Work out the finished part from the listing and answer in its coordinate system (mm). Face numbers are marked on the shaded views. A direction names the side the tool comes from. Give positions to 0.01 mm unless a question says otherwise; leave off trailing zeros. Loops run counter-clockwise (first coordinate to the right, second up) from the corner with the lowest first, then second, coordinate; pieces in that order, holes last. Notation, with made-up numbers: (75.25, 65.25) - (125.25, 65.25) arc R33 cw to (125.25, 100.25) - close; hole circle Ø8 at (38.5, -7.75). An arc over 180 degrees is marked (long way). One line per item, written item: value.
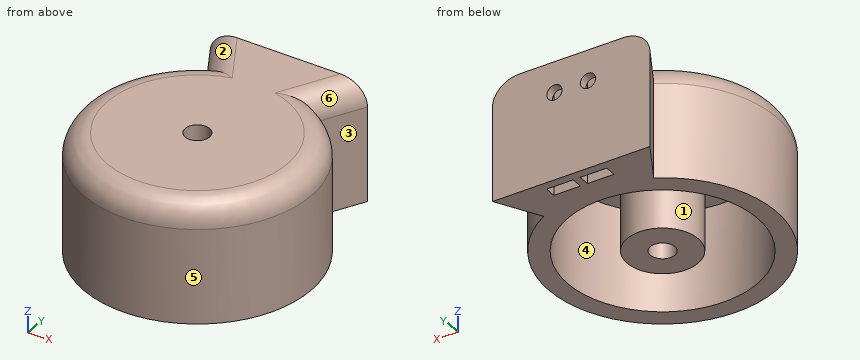
from build123d import *

# Parameters (mm, degrees)
BOSS_EXTRUDE1_DEPTH = 25
FILLET1_R           = 5
SKETCH2_R           = 2.6
CUT_EXTRUDE1_DEPTH  = 46.836666718
SKETCH4_R           = 20
SKETCH4_R_2         = 7.5
CUT_EXTRUDE2_DEPTH  = 21
CUT_EXTRUDE3_START  = 30
SKETCH5_R           = 1.6
CUT_EXTRUDE3_DEPTH  = 6
SKETCH6_W           = 5.6
SKETCH6_H           = 2.4
CUT_EXTRUDE4_DEPTH  = 22.5


with BuildPart() as part:
    # Sketch1 → Boss-Extrude1 (new body)
    with BuildSketch(Plane.XY):
        with BuildLine():
            Line((-16.642519968, 30), (16.642519968, 30))
            Line((16.642519968, 30), (11.642519968, 20.986941864))
            ThreePointArc((11.642519968, 20.986941864), (0, -24), (-11.642519968, 20.986941864))
            Line((-11.642519968, 20.986941864), (-16.642519968, 30))
        make_face()
    extrude(amount=BOSS_EXTRUDE1_DEPTH)

    # Fillet1
    fillet1_edges = [part.edges().sort_by_distance(p)[0] for p in [
        (-14.142519968, 25.493470932, 25),
    ]]
    fillet(fillet1_edges, radius=FILLET1_R)
    fillet1_2_edges = [part.edges().sort_by_distance(p)[0] for p in [
        (14.142519968, 25.493470932, 25),
    ]]
    fillet(fillet1_2_edges, radius=FILLET1_R)
    fillet1_3_edges = [part.edges().sort_by_distance(p)[0] for p in [
        (0, -24, 25),
    ]]
    fillet(fillet1_3_edges, radius=FILLET1_R - 0.0001)  # a hair under: the kernel refuses the full size

    # Sketch2 → Cut-Extrude1 (cut, through all)
    with BuildSketch(Plane.XY):
        Circle(SKETCH2_R)
    extrude(amount=CUT_EXTRUDE1_DEPTH, mode=Mode.SUBTRACT)

    # Sketch4 → Cut-Extrude2 (cut)
    with BuildSketch(Plane.XY):
        with Locations(Location((0, 0, 0), (0, 0, 180))):
            Circle(SKETCH4_R)
        with Locations(Location((0, 0, 0), (0, 0, 180))):
            Circle(SKETCH4_R_2, mode=Mode.SUBTRACT)
    extrude(amount=CUT_EXTRUDE2_DEPTH, mode=Mode.SUBTRACT)

    # Sketch5 → Cut-Extrude3 (cut)
    with BuildSketch(Plane(origin=(0, 0, 0), x_dir=(1, 0, 0), z_dir=(0, 1, 0)).offset(CUT_EXTRUDE3_START)):
        with Locations(Location((-3.55, -18.5, 0), (0, 0, 90))):
            Circle(SKETCH5_R)
        with Locations(Location((3.55, -18.5, 0), (0, 0, 90))):
            Circle(SKETCH5_R)
    extrude(amount=-CUT_EXTRUDE3_DEPTH, mode=Mode.SUBTRACT)

    # Sketch6 → Cut-Extrude4 (cut)
    with BuildSketch(Plane.XY):
        with Locations((3.55, 27)):
            Rectangle(SKETCH6_W, SKETCH6_H)
        with Locations((-3.55, 27)):
            Rectangle(SKETCH6_W, SKETCH6_H)
    extrude(amount=CUT_EXTRUDE4_DEPTH, mode=Mode.SUBTRACT)


solid = part.part
1. Section C-C (x = 0) is taken. Write down the section's boundary in (y, z).
Output:
outline: (-24, 0) - (-20, 0) - (-20, 21) - (-7.5, 21) - (-7.5, 0) - (-2.6, 0) - (-2.6, 25) - (-19, 25) arc R5 ccw to (-24, 20) - close; (2.6, 0) - (7.5, 0) - (7.5, 21) - (20, 21) - (20, 0) - (30, 0) - (30, 25) - (2.6, 25) - close
2. For the marked faces 1, 2 and 3, determine the directions among +Z, -Z, +X, -X, +Y, -Y from which every point of the face is accessible in a straight line to the end or side of a thin tool.
Output:
face 1: -Z
face 2: +Z, -X
face 3: +Z, -Z, +X
3. The mould has two halves that part along X. Classify the marked faces 4, 5 and 6: released by +X, released by -X, zero draft, split by the parting line, or undercut.
Output:
face 4: undercut
face 5: split by the parting line
face 6: released by +X
4. Find the intervals of material crossed by line 1 along X through (y, z) = (1.5, 19.75); line 2 along X through (y, z) = (3, 10); line 3 along X through (y, z) = (29.05, 18.5), in increasing order.
Output:
line 1: x = -23.95 to -19.94, -7.35 to -2.12, 2.12 to 7.35, 19.94 to 23.95
line 2: x = -23.81 to -19.77, -6.87 to 6.87, 19.77 to 23.81
line 3: x = -16.12 to -5.15, -1.95 to 1.95, 5.15 to 16.12
5. Section B-B (z = 15.5) is taken. Write down the section's boundary in (x, y), and give its area (3 significant figures).
Output:
outline: (-16.64, 30) - (-11.64, 20.99) arc R24 ccw (long way) to (11.64, 20.99) - (16.64, 30) - close; circle Ø15 at (0, 0); hole circle Ø40 at (0, 0); hole (-6.35, 25.8) - (-0.75, 25.8) - (-0.75, 28.2) - (-6.35, 28.2) - close; hole circle Ø5.2 at (0, 0); hole (0.75, 25.8) - (6.35, 25.8) - (6.35, 28.2) - (0.75, 28.2) - close
area: 889 mm²
6. Section A-A (z = 18.5) is taken. Count the separate pieces of the cut face and the enclosed holes in it, and give its area (3 significant figures).
Output:
separate pieces: 2
enclosed holes: 2
area: 866 mm²
7. Flat-ended cylindrical pins translate along their axes: pin 1 Ø0.7 at (y, z) = (26.5, 15) entering from +X; pin 2 Ø6 at (x, y) = (0.5, -16) entering from -Z; pin 3 Ø6 at (x, y) = (-7.5, -16) entering from -Z; pin 4 Ø1.6 at (x, z) = (3, 18.5) entering from +Y. Find the tip coordinate at first contact, or state that the pin passes through.
Output:
pin 1: stops at x = 14.9
pin 2: stops at z = 21
pin 3: stops at z = 0
pin 4: stops at y = 24
